The listing builds one solid part. Answer for the finished solid, in the listing's coordinates (mm). Face numbers are marked on the shaded views. Coordinates: 2 decimals unless noted, no trailing zeros. Order: outer loops, then holes, each group sorted by start corner. A loop starts at its lowest first (then second) coordinate and runs counter-clockwise, first axis right, second up. Notation, with made-up numbers: (88.25, -9.5) - (119.25, -9.5) arc R18 ccw to (119.25, 1.5) - close; hole circle Ø1 at (48, 55.5). An arc over 180 degrees is marked (long way). Use a Markdown table: item, result. Add a question column.
Item 1: The mould has two halves that part along Z. Classify the marked faces 1 and 2: released by +Z, released by -Z, zero draft, split by the parting line, or undercut.
Item 2: The part is cut by section B-B, the plane z = 0. Give the vertices of the cut face in (x, y).
Item 3: The part is cut by section D-D, the plane y = -9.5. Give the vertices of the cut face in (x, z).
Item 4: Find the intervals of material crossed by line 1 along X through (y, z) = (-14.7, 11.8); line 2 along Y through (x, z) = (2.75, 6); line 3 along Z through (x, y) = (9.25, 7.5), in increasing order.
Item 5: Flat-ended cylindrical pins translate along their axes: P1, Ø3, axis at x = -7, y = 8, coming from the +Z side; P2, Ø6, axis at y = 2.5, z = 9.5, coming from the -X side; P3, Ø5, axis at x = -1, y = 6.5, coming from the +Z side; P4, Ø10, axis at x = -3.5, y = -6, coming from the -Z side. Find the tip coordinate at first contact, or state that the pin passes through.
Item 6: The part is cut by section A-A, the plane x = 0. Give the vertices of the cut face in (y, z), then the cut area to 3 significant figures.
Item 7: The part is cut by section C-C, the plane y = -14.7. Give the vertices of the cut face in (x, z).
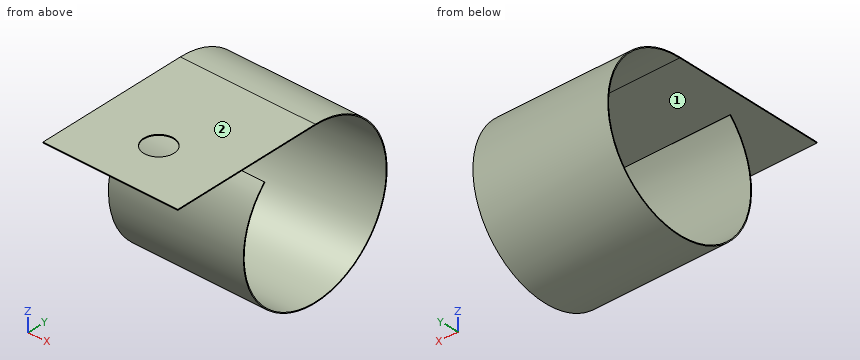
from build123d import *

# Parameters (mm, degrees)
BOSS_EXTRUDE1_DEPTH = 10
CUT_EXTRUDE1_REACH  = 36.349
SKETCH2_R           = 2.25


with BuildPart() as part:
    # Sketch1 → Boss-Extrude1 (new, symmetric)
    with BuildSketch(Plane(origin=(0, 0, 0), x_dir=(0, -1, 0), z_dir=(1, 0, 0))):
        with BuildLine():
            Line((8.40042856, -8.40042856), (8.308504679, -8.308504679))
            ThreePointArc((8.308504679, -8.308504679), (-4.49653033, 10.855584507), (0, -11.75))
            Line((0, -11.75), (22.7, -11.75))
            Line((22.7, -11.75), (22.7, -11.88))
            Line((22.7, -11.88), (0, -11.88))
            ThreePointArc((0, -11.88), (-4.546279176, 10.975688846), (8.40042856, -8.40042856))
        make_face()
    extrude(amount=BOSS_EXTRUDE1_DEPTH, both=True)

    # Sketch2 → Cut-Extrude1 (cut, up to next)
    with BuildSketch(Plane(origin=(0, 0, 11.88), x_dir=(-1, 0, 0), z_dir=(0, 0, -1)), mode=Mode.PRIVATE) as cut_extrude1_sk1:
        with Locations(Location((0, -14.7, 0), (0, 0, 180))):
            Circle(SKETCH2_R)
    cut_extrude1_tool1 = extrude(cut_extrude1_sk1.sketch, amount=CUT_EXTRUDE1_REACH, mode=Mode.PRIVATE) & part.part
    add(cut_extrude1_tool1.solids().sort_by_distance((0, -14.7, 11.88))[0], mode=Mode.SUBTRACT)


solid = part.part
Solution:
| question | item | result |
|---|---|---|
| 1 | face 1 | undercut |
| 1 | face 2 | released by +Z |
| 2 | outline | (-10, -11.88) - (10, -11.88) - (10, -11.75) - (-10, -11.75) - close; (-10, 11.75) - (10, 11.75) - (10, 11.88) - (-10, 11.88) - close |
| 3 | outline | (-10, -7.13) - (10, -7.13) - (10, -6.91) - (-10, -6.91) - close; (-10, 6.91) - (10, 6.91) - (10, 7.13) - (-10, 7.13) - close; (-10, 11.75) - (10, 11.75) - (10, 11.88) - (-10, 11.88) - close |
| 4 | line 1 | x = -10 to -2.25, 2.25 to 10 |
| 4 | line 2 | y = -10.25 to -10.1, 10.1 to 10.25 |
| 4 | line 3 | z = -9.21 to -9.05, 9.05 to 9.21 |
| 5 | P1 | stops at z = 9.94 |
| 5 | P2 | stops at x = -10 |
| 5 | P3 | stops at z = 11.19 |
| 5 | P4 | stops at z = -11.84 |
| 6 | outline | (-22.7, 11.75) - (-16.95, 11.75) - (-16.95, 11.88) - (-22.7, 11.88) - close; (-12.45, 11.75) - (0, 11.75) arc R11.75 cw (long way) to (-8.31, 8.31) - (-8.4, 8.4) arc R11.88 ccw (long way) to (0, 11.88) - (-12.45, 11.88) - close |
| 6 | area | 10.8 mm2 |
| 7 | outline | (-10, 11.75) - (-2.25, 11.75) - (-2.25, 11.88) - (-10, 11.88) - close; (2.25, 11.75) - (10, 11.75) - (10, 11.88) - (2.25, 11.88) - close |
